Design review of the part built by this model. Coordinates are the model's own, in mm. Give positions to 0.01 mm unless a question says otherwise; leave off trailing zeros. Loops run counter-clockwise (first coordinate to the right, second up) from the corner with the lowest first, then second, coordinate; pieces in that order, holes last. Notation, with made-up numbers: (-7, 82) - (13, 82) arc R30 cw to (13, 104) - close; hole circle Ø3 at (64.25, 26). An arc over 180 degrees is marked (long way). One line per item, written item: value. Start each with the question number.
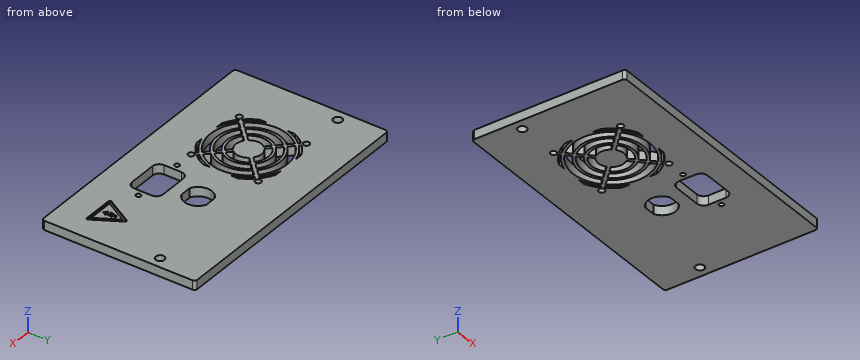
```python
from build123d import *

# Parameters (mm, degrees)
SKETCH1_W           = 200
SKETCH1_H           = 114.3
BOSS_EXTRUDE1_DEPTH = 6.8
SKETCH2_R           = 3.25
CUT_EXTRUDE1_DEPTH  = 6.8
FILLET1_R           = 2
SKETCH3_R           = 1.775
SKETCH3_W           = 31
SKETCH3_H           = 23
CUT_EXTRUDE2_DEPTH  = 6.8
FILLET2_R           = 5
SKETCH4_R           = 28.5
SKETCH4_R_2         = 23.5
SKETCH4_R_3         = 21.5
SKETCH4_R_4         = 16.5
SKETCH4_R_5         = 14.5
SKETCH4_R_6         = 9.5
SKETCH4_R_7         = 2.25
CUT_EXTRUDE3_DEPTH  = 116.379211732
BOSS_EXTRUDE7_DEPTH = 6.8
CUT_EXTRUDE6_DEPTH  = 1


with BuildPart() as part:
    # Sketch1 → Boss-Extrude1 (new body)
    with BuildSketch(Plane.XY):
        Rectangle(SKETCH1_W, SKETCH1_H)
    extrude(amount=BOSS_EXTRUDE1_DEPTH)

    # Sketch2 → Cut-Extrude1 (cut)
    with BuildSketch(Plane.XY.offset(6.8)):
        with Locations((-92, 25.25)):
            Circle(SKETCH2_R)
        with Locations((92, 25.25)):
            Circle(SKETCH2_R)
    extrude(amount=-CUT_EXTRUDE1_DEPTH, mode=Mode.SUBTRACT)

    # Fillet1
    fillet1_edges = [part.edges().sort_by_distance(p)[0] for p in [
        (-100, 57.15, 3.4),
        (100, 57.15, 3.4),
        (100, -57.15, 3.4),
        (-100, -57.15, 3.4),
    ]]
    fillet(fillet1_edges, radius=FILLET1_R)

    # Sketch3 → Cut-Extrude2 (cut)
    with BuildSketch(Plane.XY.offset(6.8)):
        with Locations((4.5, -25)):
            Circle(SKETCH3_R)
        with Locations((44.5, -25)):
            Circle(SKETCH3_R)
        with Locations((24.5, -25)):
            Rectangle(SKETCH3_W, SKETCH3_H)
        with BuildLine():
            Line((20.190417654, 14.3), (28.809582346, 14.3))
            ThreePointArc((28.809582346, 14.3), (34.75, 5), (28.809582346, -4.3))
            Line((28.809582346, -4.3), (20.190417654, -4.3))
            ThreePointArc((20.190417654, -4.3), (14.25, 5), (20.190417654, 14.3))
        make_face()
    extrude(amount=-CUT_EXTRUDE2_DEPTH, mode=Mode.SUBTRACT)

    # Fillet2
    fillet2_edges = [part.edges().sort_by_distance(p)[0] for p in [
        (40, -13.5, 3.4),
        (40, -36.5, 3.4),
        (9, -36.5, 3.4),
        (9, -13.5, 3.4),
    ]]
    fillet(fillet2_edges, radius=FILLET2_R)

    # Sketch4 → Cut-Extrude3 (cut, through all)
    with BuildSketch(Plane.XY.offset(6.8)):
        with Locations((-35, 0)):
            Circle(SKETCH4_R)
        with Locations((-35, 0)):
            Circle(SKETCH4_R_2, mode=Mode.SUBTRACT)
        with Locations((-35, 0)):
            Circle(SKETCH4_R_3)
        with Locations((-35, 0)):
            Circle(SKETCH4_R_4, mode=Mode.SUBTRACT)
        with Locations((-35, 0)):
            Circle(SKETCH4_R_5)
        with Locations((-35, 0)):
            Circle(SKETCH4_R_6, mode=Mode.SUBTRACT)
        with BuildLine():
            Line((-22.009073716, 29.55), (-27.447020455, 29.55))
            ThreePointArc((-27.447020455, 29.55), (-13.433243174, 21.566756826), (-5.45, 7.552979545))
            Line((-5.45, 7.552979545), (-5.45, 12.990926284))
            ThreePointArc((-5.45, 12.990926284), (-12.174940682, 22.825059318), (-22.009073716, 29.55))
        make_face()
        with BuildLine():
            ThreePointArc((-47.990926284, 29.55), (-57.825059318, 22.825059318), (-64.55, 12.990926284))
            Line((-64.55, 12.990926284), (-64.55, 7.552979545))
            ThreePointArc((-64.55, 7.552979545), (-56.566756826, 21.566756826), (-42.552979545, 29.55))
            Line((-42.552979545, 29.55), (-47.990926284, 29.55))
        make_face()
        with BuildLine():
            ThreePointArc((-42.552979545, -29.55), (-56.566756826, -21.566756826), (-64.55, -7.552979545))
            Line((-64.55, -7.552979545), (-64.55, -12.990926284))
            ThreePointArc((-64.55, -12.990926284), (-57.825059318, -22.825059318), (-47.990926284, -29.55))
            Line((-47.990926284, -29.55), (-42.552979545, -29.55))
        make_face()
        with BuildLine():
            ThreePointArc((-5.45, -7.552979545), (-13.433243174, -21.566756826), (-27.447020455, -29.55))
            Line((-27.447020455, -29.55), (-22.009073716, -29.55))
            ThreePointArc((-22.009073716, -29.55), (-12.174940682, -22.825059318), (-5.45, -12.990926284))
            Line((-5.45, -12.990926284), (-5.45, -7.552979545))
        make_face()
        with Locations((-10, -25)):
            Circle(SKETCH4_R_7)
        with Locations((-60, -25)):
            Circle(SKETCH4_R_7)
        with Locations((-60, 25)):
            Circle(SKETCH4_R_7)
        with Locations((-10, 25)):
            Circle(SKETCH4_R_7)
    extrude(amount=-CUT_EXTRUDE3_DEPTH, mode=Mode.SUBTRACT)


with BuildPart() as cut_extrude3_piece_1:
    # of the separate pieces the step leaves, piece 1, a body of its own (cut_extrude3_pieces)
    add(part.part.solids().sort_by_distance((98, -57.15, 0))[0])



with BuildPart() as cut_extrude3_piece_2:
    # of the separate pieces the step leaves, piece 2, a body of its own (cut_extrude3_pieces)
    add(part.part.solids().sort_by_distance((-25.5, 0, 0))[0])


with BuildPart() as cut_extrude3_piece_3:
    # of the separate pieces the step leaves, piece 3, a body of its own (cut_extrude3_pieces)
    add(part.part.solids().sort_by_distance((-11.5, 0, 0))[0])


with BuildPart() as cut_extrude3_piece_4:
    # of the separate pieces the step leaves, piece 4, a body of its own (cut_extrude3_pieces)
    add(part.part.solids().sort_by_distance((-18.5, 0, 0))[0])


with BuildPart() as cut_extrude3_piece_1_1:
    add(cut_extrude3_piece_1.part)

    add(cut_extrude3_piece_2.part)  # Boss-Extrude7 merges Cut-Extrude3 piece 2

    add(cut_extrude3_piece_3.part)  # Boss-Extrude7 merges Cut-Extrude3 piece 3

    add(cut_extrude3_piece_4.part)  # Boss-Extrude7 merges Cut-Extrude3 piece 4
    # Sketch9 → Boss-Extrude7 (add)
    with BuildSketch(Plane.XY.offset(6.8)):
        Polygon((-31.982233047, 1.25), (-10.843604319, 22.388628728), (-12.611371272, 24.156395681), (-33.75, 3.017766953), (-33.75, 1.25), align=None)
        Polygon((-10.923846691, -22.308386356), (-31.982233047, -1.25), (-33.75, -1.25), (-33.75, -3.017766953), (-12.691613644, -24.076153309), align=None)
        Polygon((-36.25, 1.25), (-36.25, 3.017766953), (-57.308386356, 24.076153309), (-59.076153309, 22.308386356), (-38.017766953, 1.25), align=None)
        Polygon((-57.388628728, -24.156395681), (-36.25, -3.017766953), (-36.25, -1.25), (-38.017766953, -1.25), (-59.156395681, -22.388628728), align=None)
    extrude(amount=-BOSS_EXTRUDE7_DEPTH)

    # Sketch6 → Cut-Extrude6 (cut)
    with BuildSketch(Plane.XY.offset(6.8)):
        with BuildLine():
            Line((83.545946103, -34.5), (72.287615854, -15))
            ThreePointArc((72.287615854, -15), (71.42159045, -14.5), (70.555565047, -15))
            Line((70.555565047, -15), (59.297234797, -34.5))
            ThreePointArc((59.297234797, -34.5), (59.297234797, -35.5), (60.163260201, -36))
            Line((60.163260201, -36), (82.6799207, -36))
            ThreePointArc((82.6799207, -36), (83.545946103, -35.5), (83.545946103, -34.5))
        make_face()
        Polygon((61.895311009, -34), (80.947869892, -34), (71.42159045, -17.5), align=None, mode=Mode.SUBTRACT)
        Polygon((69.142579413, -27.8405455), (70.551015324, -22.149276649), (72.347394106, -22.149276649), (71.107138719, -25.764726734), (73.151026627, -24.109810005), (72.107844017, -29.983919065), (73.346390955, -28.98107931), (71.626753961, -32.031548417), (69.423161567, -29.310024263), (70.811409093, -30.092619241), (71.42159045, -26.709391164), align=None)
    extrude(amount=-CUT_EXTRUDE6_DEPTH, mode=Mode.SUBTRACT)


solid = cut_extrude3_piece_1_1.part
```
(1) Take a section at A-A on x = -92. State the section outline as (y, z) points.
(2) Take a section at B-B on z = 2. State how many separate pieces and enclosed holes the cut face has, and give its area (3 significant figures).
(3) To check wall thickness, follow L1, parallel to Y at x = -10, z = 2.5; L2, parallel to Y at x = 4.5, z = 3.25 (3 decimals); L3, parallel to Y at x = -52, z = 5.25. State the ranges of each line that lie inside material, in increasing order. Write a range as from..to.
Here are the results:
1. outline: (-57.15, 0) - (22, 0) - (22, 6.8) - (-57.15, 6.8) - close; (28.5, 0) - (57.15, 0) - (57.15, 6.8) - (28.5, 6.8) - close
2. separate pieces: 1
2. enclosed holes: 30
2. area: 19,900 mm²
3. L1: -57.15..-27.25, -22.75..-20.42, -17.47..-13.68, 13.68..17.47, 20.42..22.75, 27.25..57.15
3. L2: -57.15..-26.775, -23.225..57.15
3. L3: -57.15..-27.44, -25.32..-22.87, -18.77..-13.16, 13.16..18.77, 22.87..25.32, 27.44..57.15
